Verification items for the finished model (mm, model axes). A direction names the side the tool comes from. Give positions to 0.01 mm unless a question says otherwise; leave off trailing zeros. Write each loop counter-clockwise with the first axis right and the second up, starting at its lowest first coordinate (ties: lowest second). Pieces come first, ordered by that corner, then holes. Notation, with made-up numbers: (46.25, 26.25) -> (69.25, 26.25) arc R32 cw to (69.25, 63.25) -> close; hole circle Ø10 at (39.5, 20.25). An arc over 180 degrees is marked (long way). Use one line per item in the form item = value. Start each with the question number.
(1) Depth check by flat-ended pin: pin 1 Ø10 at (x, y) = (117, 36) entering from +Z. Enter the tip coordinate at first touch or a pass-through.
(2) Release check for a two-part mould opening along X. For faces 3 (the face through (92, 42, 0)), 4 (the face through (187.5, 41, 5)), 5 (the face through (95, 77.5, 7)), 6 (the face through (182.5, 41, 7)) record: pulls with the +X half, pulls with the -X half, needs draft (parallel to the pull), parting line crosses it, or undercut.
(3) Section check C-C, the plane x = 85.5. Record the cut outline in (y, z).
(4) Set-up check for faces 1 (the face through (93, 5, 7)), 2 (the face through (95, 82.5, 5)): record each of +Z, -Z, +X, -X, +Y, -Y from which the full face is reachable in a straight line by a thin tool's end or side.
(5) Section check A-A, the plane z = 5.5. Record the cut outline in (x, y), plus the area to 3 significant figures.
(6) Scan lines: L1, parallel to Y at x = 116, z = 3.25; L2, parallel to X at y = 43, z = 6.5; L3, parallel to Z at x = 85, y = 48. Record each from-to range of solid material in increasing order.
(7) Section check B-B, the plane y = 25. Record the cut outline in (x, z), plus the area to 4 significant figures.
Autodesk Fusion 360 part; units mm, degrees
sketch "Sketch1" plane through (0, 0, 0) normal (0, 0, 1) x (1, 0, 0)
  line L0 (0, 0) -> (187.5, 0)
  line L1 (187.5, 0) -> (187.5, 82.5)
  line L2 (187.5, 82.5) -> (0, 82.5)
  line L3 (0, 82.5) -> (0, 0)
  dimension "d1" = 187.5
  dimension "d2" = 82.5
extrude "Extrude1" add sketch "Sketch1" along normal blind 3
sketch "Sketch2" plane through (0, 0, 3) normal (0, 0, 1) x (-1, 0, 0)
  line L0 (0, -82.5) -> (0, 0)
  line L1 (0, 0) -> (-187.5, 0)
  line L2 (-187.5, 0) -> (-187.5, -82.5)
  line L3 (-187.5, -82.5) -> (0, -82.5)
  line L4 (-5, -5) -> (-182.5, -5)
  line L5 (-182.5, -5) -> (-182.5, -77.5)
  line L6 (-182.5, -77.5) -> (-5, -77.5)
  line L7 (-5, -77.5) -> (-5, -5)
  dimension "d5" = -5
extrude "Extrude2" add sketch "Sketch2" along normal blind 8
Completed:
q1.pin_1 = 3
q2.face_3 = needs draft
q2.face_4 = pulls with the +X half
q2.face_5 = undercut
q2.face_6 = undercut
q3.outline = (0, 0) -> (82.5, 0) -> (82.5, 11) -> (77.5, 11) -> (77.5, 3) -> (5, 3) -> (5, 11) -> (0, 11) -> close
q4.face_1 = +Z
q4.face_2 = +Z, -Z, +X, -X, +Y
q5.outline = (0, 0) -> (187.5, 0) -> (187.5, 82.5) -> (0, 82.5) -> close; hole (5, 5) -> (182.5, 5) -> (182.5, 77.5) -> (5, 77.5) -> close
q5.area = 2,600 mm²
q6.L1 = 0 to 5, 77.5 to 82.5
q6.L2 = 0 to 5, 182.5 to 187.5
q6.L3 = 0 to 3
q7.outline = (0, 0) -> (187.5, 0) -> (187.5, 11) -> (182.5, 11) -> (182.5, 3) -> (5, 3) -> (5, 11) -> (0, 11) -> close
q7.area = 642.5 mm²
